The model under review builds one solid part; all positions refer to its coordinate system, in mm. Face numbers are marked on the shaded views. A direction names the side the tool comes from. Round coordinates to 2 decimals unless told otherwise and drop trailing zeros. Write each loop counter-clockwise with the first axis right and the second up, starting at its lowest first coordinate (ties: lowest second). Pieces come first, ordered by that corner, then holes. Notation, with made-up numbers: (-6.5, -23) - (36.5, -23) arc R17 ccw to (36.5, -14) - close; hole circle Ø1 at (35, 73). An arc over 180 degrees is marked (long way). Return JSON: item names as keys, results as strings.
from build123d import *

# Parameters (mm, degrees)
SKETCH2_W           = 6.35
SKETCH2_H           = 6.35
BOSS_EXTRUDE1_DEPTH = 40.64
BOSS_EXTRUDE2_DEPTH = 2.54


with BuildPart() as part:
    # Sketch2 → Boss-Extrude1 (new body)
    with BuildSketch(Plane(origin=(0, 0, 0), x_dir=(1, 0, 0), z_dir=(0, 1, 0))):
        Polygon((-33.02, 0), (0, 0), (0, 21.082), (0, 27.432), (0, 34.29), (-16.51, 21.59), (-33.02, 34.29), (-33.02, 27.432), (-33.02, 21.082), align=None)
        with Locations((-36.195, 24.257)):
            Rectangle(SKETCH2_W, SKETCH2_H)
        with Locations((3.175, 24.257)):
            Rectangle(SKETCH2_W, SKETCH2_H)
    extrude(amount=BOSS_EXTRUDE1_DEPTH)

    # Sketch5 → Boss-Extrude2 (add)
    with BuildSketch(Plane.XZ):
        Polygon((0, -34.29), (-33.02, -34.29), (-16.51, -21.59), align=None)
    extrude(amount=-BOSS_EXTRUDE2_DEPTH)


solid = part.part
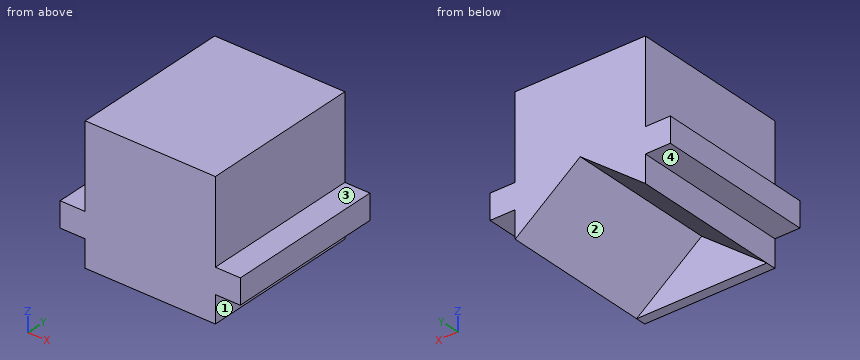
(1) Add section A-A (x = -13). Write out the cut boundary in (y, z).
Filled in:
{"outline": "(0, -34.29) - (2.54, -34.29) - (2.54, -24.29) - (40.64, -24.29) - (40.64, 0) - (0, 0) - close"}
(2) Add section D-D (z = -23). Write out the cut boundary in (x, y).
Filled in:
{"outline": "(-39.37, 0) - (6.35, 0) - (6.35, 40.64) - (-14.68, 40.64) - (-14.68, 2.54) - (-18.34, 2.54) - (-18.34, 40.64) - (-39.37, 40.64) - close"}
(3) Add section B-B (y = 11). Write out the cut boundary in (x, z), plus the area to 3 significant figures.
Filled in:
{"outline": "(-39.37, -27.43) - (-33.02, -27.43) - (-33.02, -34.29) - (-16.51, -21.59) - (0, -34.29) - (0, -27.43) - (6.35, -27.43) - (6.35, -21.08) - (0, -21.08) - (0, 0) - (-33.02, 0) - (-33.02, -21.08) - (-39.37, -21.08) - close", "area": "1,000 mm2"}
(4) Clearance check with flat-ended pins moving along their axes: pin 1 Ø10 at (y, z) = (25, -6) entering from +X; pin 2 Ø2 at (x, y) = (-27.5, 27) entering from -Z; pin 3 Ø6.5 at (x, z) = (-16.5, -27.5) entering from +Y. State where each tip first meets the part, or that it passes through.
Filled in:
{"pin 1": "stops at x = 0", "pin 2": "stops at z = -30.81", "pin 3": "stops at y = 2.54"}
(5) Add section C-C (z = -29.5). Write out the cut boundary in (x, y), plus the area to 3 significant figures.
Filled in:
{"outline": "(-33.02, 0) - (0, 0) - (0, 40.64) - (-6.23, 40.64) - (-6.23, 2.54) - (-26.79, 2.54) - (-26.79, 40.64) - (-33.02, 40.64) - close", "area": "558 mm2"}
(6) Wall thickness on line 1 (X direction, y = 24, z = -17); line 2 (X direction, y = 25, z = -22); line 3 (X direction, y = 27, z = -29): over which ranges is each line inside the solid? List them lowest first.
Filled in:
{"line 1": "x = -33.02 to 0", "line 2": "x = -39.37 to -17.04, -15.98 to 6.35", "line 3": "x = -33.02 to -26.14, -6.88 to 0"}
(7) For the marked faces 1, 2, 3 and 4, list the 3-axis set-ups (+Z, -Z, +X, -X, +Y, -Y) from which the entire face can be reached by the end or side of a thin tool; tool diameter is ignored.
Filled in:
{"face 1": "-Z, +X, +Y, -Y", "face 2": "-Z, +Y", "face 3": "+Z, +X, +Y, -Y", "face 4": "-Z, -X, +Y, -Y"}
